from build123d import *

# Parameters (mm, degrees)
BOSS_EXTRUDE1_DEPTH = 0.889
SKETCH2_R           = 5.3975
SKETCH2_R_2         = 3.6195
BOSS_EXTRUDE2_DEPTH = 0.889
SKETCH3_W           = 10.16
SKETCH3_H           = 10.16
SKETCH3_W_2         = 6.604
SKETCH3_H_2         = 6.604
BOSS_EXTRUDE3_DEPTH = 0.889
SKETCH4_R           = 0.762
BOSS_EXTRUDE4_START = -2.54
SKETCH8_R           = 0.00127
BOSS_EXTRUDE4_DEPTH = 18.999523


with BuildPart() as part:
    # Sketch1 → Boss-Extrude1 (new body, symmetric)
    with BuildSketch(Plane.XY):
        Polygon((0, 0), (-6.35, -10.998522628), (6.35, -10.998522628), align=None)
        Polygon((0, -3.556), (-3.270413664, -9.220522628), (3.270413664, -9.220522628), align=None, mode=Mode.SUBTRACT)
    extrude(amount=BOSS_EXTRUDE1_DEPTH, both=True)

    # Sketch4 → Revolve1 (revolve)
    with BuildSketch(Plane.XY):
        with Locations((0, -1.524)):
            Circle(SKETCH4_R)
    revolve(axis=Axis((0, 0.254, 0), (1, 0, 0)))

    # Sketch5 → Cut-Revolve1 (revolve, cut)
    with BuildSketch(Plane.XY):
        with BuildLine():
            Line((-0.659911358, -1.143), (-0.659911358, 0.254))
            Line((-0.659911358, 0.254), (0.659911358, 0.254))
            Line((0.659911358, 0.254), (0.659911358, -1.143))
            ThreePointArc((0.659911358, -1.143), (0, -0.762), (-0.659911358, -1.143))
        make_face()
    revolve(axis=Axis((0.659911358, 0.254, 0), (-1, 0, 0)), mode=Mode.SUBTRACT)



with BuildPart() as body_2:
    # Sketch2 → Boss-Extrude2 (new body, symmetric)
    with BuildSketch(Plane(origin=(0, 0, 0), x_dir=(0, 0, -1), z_dir=(1, 0, 0))):
        with Locations((0, -12.078022628)):
            Circle(SKETCH2_R)
        with Locations((0, -12.078022628)):
            Circle(SKETCH2_R_2, mode=Mode.SUBTRACT)
    extrude(amount=BOSS_EXTRUDE2_DEPTH, both=True)


with BuildPart() as body_3:
    # Sketch3 → Boss-Extrude3 (new body, symmetric)
    with BuildSketch(Plane.XY):
        with Locations((0, -18.237522628)):
            Rectangle(SKETCH3_W, SKETCH3_H)
        with Locations((0, -18.237522628)):
            Rectangle(SKETCH3_W_2, SKETCH3_H_2, mode=Mode.SUBTRACT)
    extrude(amount=BOSS_EXTRUDE3_DEPTH, both=True)


with BuildPart() as part_1:
    add(part.part)

    add(body_2.part)  # Boss-Extrude4 merges body 2

    add(body_3.part)  # Boss-Extrude4 merges body 3
    # Sketch8 → Boss-Extrude4 (add)
    with BuildSketch(Plane(origin=(0, 0, 0), x_dir=(1, 0, 0), z_dir=(0, 1, 0)).offset(BOSS_EXTRUDE4_START)):
        Circle(SKETCH8_R)
    extrude(amount=-BOSS_EXTRUDE4_DEPTH)


solid = part_1.part
Geometry check sheet. Reference: the model listing, model coordinates, mm. A direction names the side the tool comes from. Round coordinates to 2 decimals unless told otherwise and drop trailing zeros. Loops run counter-clockwise (first coordinate to the right, second up) from the corner with the lowest first, then second, coordinate; pieces in that order, holes last.
Item 1: Access from +Z, -Z, +X, -X, +Y, -Y to the whole of each face (thin tool, end or side, straight path). Record for faces 5 (the flat face through (5.08, -18, 0)), 6 (the flat face through (-5.08, -18, 0)), 7 (the flat face through (-3.302, -18, 0)).
Item 2: Gauge pin test, flat ends, axial feed: pin 1 (5 mm diameter, centred on x = 1, y = -19, fed in from +Z); pin 2 (0.5 mm diameter, centred on x = -1.5, z = 0, fed in from +Y); pin 3 (0.5 mm diameter, centred on y = -17.5, z = 0.5, fed in from +X); pin 4 (6 mm diameter, centred on y = -12.08, z = 0, fed in from -X). Record the tip position at first contact, or that the pin passes through.
Item 3: Cross-section at D-D on z = -4.5. Record the boundary of the cut face in (x, y), then the cut area to 3 significant figures.
Item 4: Cross-section at B-B on z = 0.25. Count the separate pieces of the cut face and the enclosed holes in it, then the cut area to 3 significant figures.
Item 5: Thickness scan on line 1 (Z direction, x = 4, y = -21.5); line 2 (Y direction, x = 2.75, z = -0.5); line 3 (Y direction, x = -3.5, z = -0.25). Record the ranges inside material, lowest first.
Item 6: Mould release check, pull along X, two halves, no side actions. Record for faces 1 (the flat face through (0, -21.54, 0.2)), 2 (the flat face through (-3.465, -6.002, 0.012)), 3 (the flat face through (-0.1, -10.999, 0.2)), 4 (the flat face through (3.302, -18, 0)): pulls with the +X half, pulls with the -X half, needs draft (parallel to the pull), parting line crosses it, or undercut.
Answer sheet:
1. face 5: +Z, -Z, +X, -Y
1. face 6: +Z, -Z, -X, -Y
1. face 7: +Z, -Z
2. pin 1: stops at z = 3.09
2. pin 2: stops at y = -2.17
2. pin 3: stops at x = 5.08
2. pin 4: stops at x = -6.35
3. outline: (-0.89, -15.06) - (0.89, -15.06) - (0.89, -9.1) - (-0.89, -9.1) - close
3. area: 10.6 mm2
4. separate pieces: 5
4. enclosed holes: 2
4. area: 119 mm2
5. line 1: z = -0.89 to 0.89
5. line 2: y = -23.32 to -21.54, -14.94 to -13.16, -11 to -9.22, -8.32 to -4.76
5. line 3: y = -23.32 to -13.16, -11 to -6.06
6. face 1: undercut
6. face 2: pulls with the -X half
6. face 3: needs draft
6. face 4: undercut
